Verification items for the finished model (mm, model axes). Face numbers are marked on the shaded views. A direction names the side the tool comes from. Coordinates: 2 decimals unless noted, no trailing zeros. Order: outer loops, then holes, each group sorted by start corner. A loop starts at its lowest first (then second) coordinate and runs counter-clockwise, first axis right, second up. Notation, with made-up numbers: (36.5, 65.25) -> (69.5, 65.25) arc R30 cw to (69.5, 94.25) -> close; hole circle Ø7 at (55, 68). An arc over 180 degrees is marked (long way). Write each question's results on one line, items separated by ' | '. Start each with the question number.
(1) Cross-section at C-C on z = 2. Enter the section's corners in (x, y).
(2) Thickness scan on probe 1 along Z at (x, y) = (0, -14.25); probe 2 along X at (y, z) = (-6.5, 3.25); probe 3 along Y at (x, z) = (19.5, -2.5). Record the ranges inside material, lowest first. Write a range as [from, to].
(3) Cross-section at B-B on z = -6. Enter the section's corners in (x, y), and give its area (4 significant figures).
(4) Set-up check for the marked faces 1, 2, 3, 4 and 5: record each of +Z, -Z, +X, -X, +Y, -Y from which the full face is reachable in a straight line by a thin tool's end or side.
(5) Cross-section at A-A on x = 0. Enter the section's corners in (y, z), and give its area (3 significant figures).
(6) Go/stop test with flat-tipped pins: pin 1 (8 mm diameter, centred on x = -5.5, y = -4.5, fed in from +Z); pin 2 (1.5 mm diameter, centred on x = 10, y = -19.5, fed in from +Z); pin 3 (2 mm diameter, centred on x = -9.5, y = -24.5, fed in from +Z); pin 4 (2.5 mm diameter, centred on y = -9.5, z = 3.5, fed in from +X). Record where each tip stops, or that it passes through.
```python
from build123d import *

# Parameters (mm, degrees)
F1_DEPTH = 25
F2_W     = 45
F2_H     = 2
F3_DEPTH = 8
F4_R     = 2.5
F5_DEPTH = 25.0010001


with BuildPart() as f1:
    # F0 (on Front) → F1 (new body)
    with BuildSketch(Plane.XZ):
        with BuildLine():
            Line((2.5, 8), (-2.5, 8))
            Line((-2.5, 8), (-2.5, 0))
            add(Edge.make_bspline(
                [(-22.5, -5), (-19.3471894975, -4.5721768041), (-11.550922006, -4.5818809698), (-4.9118634705, -1.4177504321), (-2.5, 0)],
                knots=[0, 0, 0, 0, 0.5120347551, 1, 1, 1, 1], degree=3))
            Line((-22.5, -5), (-22.5, -8))
            Line((-22.5, -8), (-2.5, -8))
            Line((-2.5, -8), (2.5, -8))
            Line((2.5, -8), (22.5, -8))
            Line((22.5, -8), (22.5, -5))
            add(Edge.make_bspline(
                [(22.5, -5), (19.3471894975, -4.5721768041), (11.550922006, -4.5818809698), (4.9118634705, -1.4177504321), (2.5, 0)],
                knots=[0, 0, 0, 0, 0.5120347551, 1, 1, 1, 1], degree=3))
            Line((2.5, 0), (2.5, 8))
        make_face()
    extrude(amount=F1_DEPTH)

    # F2 (on Top) → F3 (join)
    with BuildSketch(Plane.XY):
        with Locations((0, -24)):
            Rectangle(F2_W, F2_H)
    extrude(amount=-F3_DEPTH)

    # F4 (on face) → F5 (cut, through all)
    with BuildSketch(Plane.XZ.offset(25)):
        with Locations((0, -4.5)):
            Circle(F4_R)
    extrude(amount=-F5_DEPTH, mode=Mode.SUBTRACT)


solid = f1.part
```
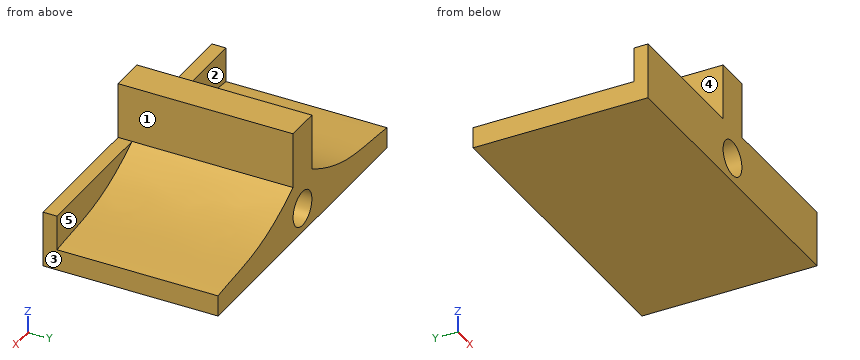
Results are:
1) outline: (-2.5, -25) -> (2.5, -25) -> (2.5, 0) -> (-2.5, 0) -> close
2) probe 1: z = [-8, -7], [-2, 8] | probe 2: x = [-2.5, 2.5] | probe 3: y = [-25, -23]
3) outline: (-22.5, -25) -> (-2, -25) -> (-2, 0) -> (-22.5, 0) -> close; (2, -25) -> (22.5, -25) -> (22.5, 0) -> (2, 0) -> close | area: 1,025 mm2
4) face 1: +Z, +X, +Y, -Y | face 2: +Z, -X, +Y | face 3: +Z, -Z, +X, +Y, -Y | face 4: +Z, -X, +Y, -Y | face 5: +Z, +X, +Y
5) outline: (-25, -8) -> (0, -8) -> (0, -7) -> (-25, -7) -> close; (-25, -2) -> (0, -2) -> (0, 8) -> (-25, 8) -> close | area: 275 mm2
6) pin 1: stops at z = 8 | pin 2: stops at z = -3.08 | pin 3: stops at z = 0 | pin 4: stops at x = 2.5
